```python
from build123d import *

# Parameters (mm, degrees)
PAD_DEPTH    = 20
SKETCH001_W  = 3
SKETCH001_H  = 10
POCKET_DEPTH = 8.501
FILLET_R     = 4.5


with BuildPart() as part:
    # Sketch → Pad (new body)
    with BuildSketch(Plane.XY):
        Polygon((-7, 2.5), (-7, -2.5), (0, -2.5), (0, -6), (10, -6), (10, 6), (0, 6), (0, 2.5), align=None)
    extrude(amount=PAD_DEPTH)

    # Sketch001 (on DatumPlane) → Pocket (cut, through all)
    with BuildSketch(Plane.XZ.offset(2.5)):
        with Locations((-1.5, 5)):
            Rectangle(SKETCH001_W, SKETCH001_H)
    extrude(amount=-POCKET_DEPTH, mode=Mode.SUBTRACT)

    # Fillet
    fillet_edges = [part.edges().sort_by_distance(p)[0] for p in [
        (10, 6, 10),
        (10, -6, 10),
    ]]
    fillet(fillet_edges, radius=FILLET_R)


solid = part.part
```
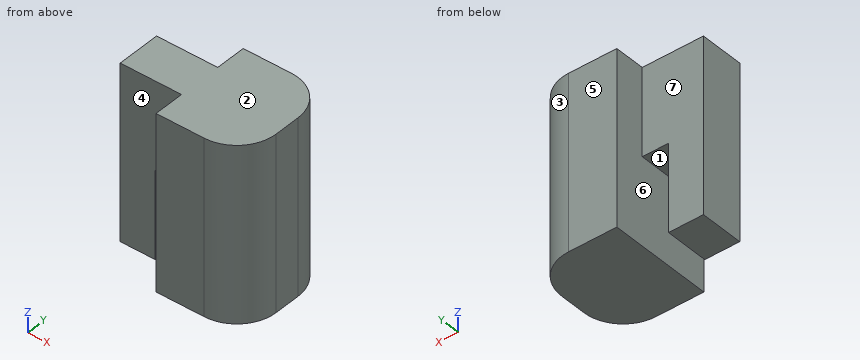
Geometry check sheet. Reference: the model listing, model coordinates, mm. Face numbers are marked on the shaded views. A direction names the side the tool comes from. Round coordinates to 2 decimals unless told otherwise and drop trailing zeros. Loops run counter-clockwise (first coordinate to the right, second up) from the corner with the lowest first, then second, coordinate; pieces in that order, holes last. Notation, with made-up numbers: (31.25, 13) - (72.25, 13) arc R13 cw to (72.25, 19) - close; hole circle Ø1 at (-35, -25). An arc over 180 degrees is marked (long way). Write item = value, one per line. Start each with the question number.
1. Section check B-B on y = 2.25. Enter the section's corners in (x, z).
2. Section check D-D on x = -1. Enter the section's corners in (y, z).
3. Depth check by flat-ended pin: pin 1 (5.5 mm diameter, centred on x = -2, z = 13.5, fed in from +Y); pin 2 (1.5 mm diameter, centred on y = -5, z = 10.5, fed in from -X); pin 3 (2 mm diameter, centred on y = 3, z = 11.5, fed in from +X). Enter the tip coordinate at first touch or a pass-through.
4. Mould release check, pull along X, two halves, no side actions. Record for the marked faces 1, 2 and 3: released by +X, released by -X, zero draft, split by the parting line, or undercut.
5. Section check C-C on z = 16.5. Enter the section's corners in (x, y).
6. Section check A-A on z = 1.5. Enter the section's corners in (x, y), then the cut area to 3 significant figures.
7. Thickness scan on line 1 (Y direction, x = -1.25, z = 14); line 2 (X direction, y = -2, z = 7); line 3 (X direction, y = 2, z = 16.25). Record the ranges inside material, lowest first.
8. Set-up check for the marked faces 4, 5, 6 and 7: record each of +Z, -Z, +X, -X, +Y, -Y from which the full face is reachable in a straight line by a thin tool's end or side.
Working result:
q1.outline = (-7, 0) - (-3, 0) - (-3, 10) - (0, 10) - (0, 0) - (9.94, 0) - (9.94, 20) - (-7, 20) - close
q2.outline = (-2.5, 10) - (2.5, 10) - (2.5, 20) - (-2.5, 20) - close
q3.pin_1 = 6
q3.pin_2 = 0
q3.pin_3 = 9.97
q4.face_1 = undercut
q4.face_2 = zero draft
q4.face_3 = released by +X
q5.outline = (-7, -2.5) - (0, -2.5) - (0, -6) - (5.5, -6) arc R4.5 ccw to (10, -1.5) - (10, 1.5) arc R4.5 ccw to (5.5, 6) - (0, 6) - (0, 2.5) - (-7, 2.5) - close
q6.outline = (-7, -2.5) - (-3, -2.5) - (-3, 2.5) - (-7, 2.5) - close; (0, -6) - (5.5, -6) arc R4.5 ccw to (10, -1.5) - (10, 1.5) arc R4.5 ccw to (5.5, 6) - (0, 6) - close
q6.area = 131 mm^2
q7.line_1 = -2.5 to 2.5
q7.line_2 = -7 to -3, 0 to 9.97
q7.line_3 = -7 to 9.97
q8.face_4 = +Z, -Z, -X, -Y
q8.face_5 = +Z, -Z, +X, -X, +Y
q8.face_6 = -Z
q8.face_7 = +Z, -Z, -X, +Y
